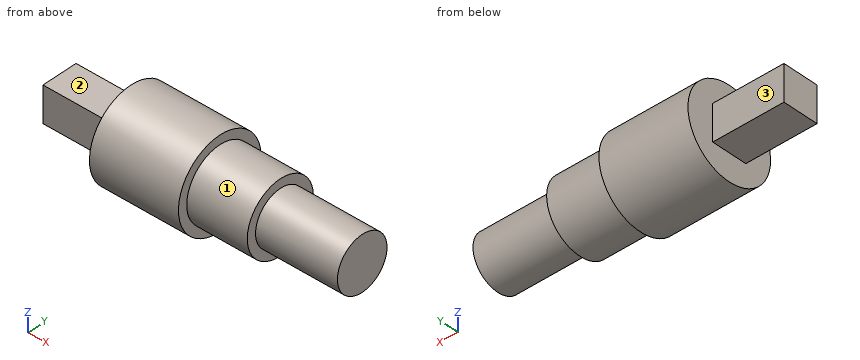
from build123d import *

# Parameters (mm, degrees)
SKETCH_3_W      = 10
SKETCH_3_H      = 10
EXTRUDE_1_DEPTH = 20


with BuildPart() as part:
    # Эскиз2 → Повернуть1 (revolve)
    with BuildSketch(Plane.XY, mode=Mode.PRIVATE) as revolve_1_sk:
        Polygon((0, 0), (0, 5), (20, 5), (20, 12.5), (45, 12.5), (45, 10), (62, 10), (62, 7.5), (85, 7.5), (85, 0), align=None)
    revolve(revolve_1_sk.sketch.rotate(Axis((0, 0, 0), (1, 0, 0)), 90), axis=Axis((0, 0, 0), (1, 0, 0)))

    # Эскиз3 → Бобышка-Вытянуть1 (add)
    with BuildSketch(Plane.ZY):
        Rectangle(SKETCH_3_W, SKETCH_3_H)
    extrude(amount=-EXTRUDE_1_DEPTH)


solid = part.part
Geometry: final body of the model. Coordinates: model frame, mm. Face numbers are marked on the shaded views. A direction names the side the tool comes from. Give positions to 0.01 mm unless a question says otherwise; leave off trailing zeros. Write each loop counter-clockwise with the first axis right and the second up, starting at its lowest first coordinate (ties: lowest second). Pieces come first, ordered by that corner, then holes.
(1) Ray query, line 1 (X direction, y = -8.5, z = -1.75); line 2 (X direction, y = 9.75, z = 4.75); line 3 (Z direction, x = 17, y = 2). Return the intervals inside material, ascending.
(2) Access query for the marked faces 1, 2 and 3. Directions: +Z, -Z, +X, -X, +Y, -Y. A direction counts if a zero-diameter tool reaches every point of the face in a straight line with its end or side. Return the directions, or none.
(3) First-contact query: P1, Ø12.5, axis at y = -1.5, z = 3.5, coming from the -X side; P2, Ø3, axis at x = 15, y = 2, coming from the +Z side; P3, Ø2, axis at x = 76, z = -3, coming from the +Y side; P4, Ø8, axis at x = 10, z = 2, coming from the -Y side. Flat tips, straight axial feed; report the tip coordinate or a pass-through.
(4) Cut plane D-D, the plane x = 73. Return loops of the section in (y, z), then the cut area to 3 significant figures.
(5) Cut plane C-C, the plane x = 33. Return loops of the section in (y, z).
(6) Cut plane A-A, the plane z = 0. Return loops of the section in (x, y).
Values follow:
1. line 1: x = 20 to 62
1. line 2: x = 20 to 45
1. line 3: z = -5 to 5
2. face 1: +X
2. face 2: +Z, -X, +Y, -Y
2. face 3: +Z, -Z, -X, +Y
3. P1: stops at x = 0
3. P2: stops at z = 5
3. P3: stops at y = 7.23
3. P4: stops at y = -5
4. outline: circle Ø15 at (0, 0)
4. area: 177 mm2
5. outline: circle Ø25 at (0, 0)
6. outline: (0, -5) - (20, -5) - (20, -12.5) - (45, -12.5) - (45, -10) - (62, -10) - (62, -7.5) - (85, -7.5) - (85, 7.5) - (62, 7.5) - (62, 10) - (45, 10) - (45, 12.5) - (20, 12.5) - (20, 5) - (0, 5) - close
